Autodesk Inventor part; units mm, degrees
ref_plane "YZ Plane" through (0, 0, 0) normal (1, 0, 0) x (0, 1, 0)
ref_plane "XZ Plane" through (0, 0, 0) normal (0, 1, 0) x (-1, 0, 0)
ref_plane "XY Plane" through (0, 0, 0) normal (0, 0, 1) x (1, 0, 0)
sketch "Sketch1" plane through (0, 0, 0) normal (0, 1, 0) x (-1, 0, 0)
  line L0 (-112.5, 75) -> (112.5, 75)
  line L1 (112.5, 75) -> (112.5, -75)
  line L2 (112.5, -75) -> (-112.5, -75)
  line L3 (-112.5, -75) -> (-112.5, 75)
  line L4 (-112.5, 75) -> (112.5, -75) construction
  line L5 (112.5, 75) -> (-112.5, -75) construction
  point P0 (0, 0)
  dimension "d0" = 225
  dimension "d1" = 150
extrude "Extrusion1" add sketch "Sketch1" along normal blind 10
sketch "Sketch2" plane through (112.5, 0, 75) normal (1, 0, 0) x (0, 0, -1)
  line L0 (0, 2.5) -> (150, 2.5)
  line L1 (150, 2.5) -> (150, 7.5)
  line L2 (150, 7.5) -> (0, 7.5)
  line L3 (0, 7.5) -> (0, 2.5)
  point P0 (75, 0)
  point P1 (0, 5)
  dimension "d4" = 150
  dimension "d5" = 5
extrude "Extrusion2" add sketch "Sketch2" along normal blind 10
sketch "Sketch3" plane through (-112.5, 0, 75) normal (0, 0, 1) x (1, 0, 0)
  line L0 (0, 2.5) -> (225, 2.5)
  line L1 (225, 2.5) -> (225, 7.5)
  line L2 (225, 7.5) -> (0, 7.5)
  line L3 (0, 7.5) -> (0, 2.5)
  point P0 (112.5, 0)
  dimension "d8" = 225
  dimension "d9" = 5
extrude "Extrusion3" add sketch "Sketch3" along normal blind 10
sketch "Sketch4" plane through (-112.5, 7.5, 75) normal (0, 1, 0) x (1, 0, 0)
  line L0 (0, -10) -> (225, -10)
  line L1 (225, -10) -> (215, -10)
  line L2 (215, -10) -> (215, 0)
  line L3 (215, 0) -> (225, 0)
  line L4 (225, 0) -> (225, -10)
  line L5 (235, 150) -> (235, 0)
  line L6 (235, 0) -> (225, 0)
  line L7 (225, 0) -> (225, 10)
  line L8 (225, 10) -> (235, 10)
  line L9 (235, 10) -> (235, 0)
  point P0 (112.5, 75)
  dimension "d12" = 10
  dimension "d13" = 10
  dimension "d14" = 10
  dimension "d15" = 10
extrude "Extrusion4" cut sketch "Sketch4" against normal blind 10
properties part number "TSU_Baseplate_Male_Cut"
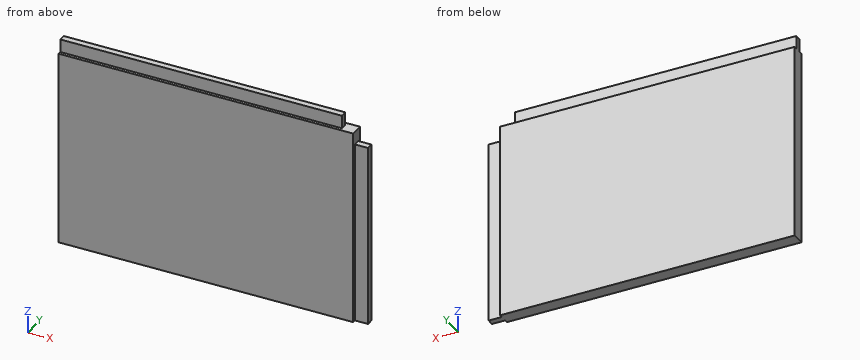
Model file for the job. Use its own axes, mm. Coordinates: 2 decimals unless noted, no trailing zeros. Loops run counter-clockwise (first coordinate to the right, second up) from the corner with the lowest first, then second, coordinate; pieces in that order, holes last. Notation, with made-up numbers: (44, 13.5) -> (57, 13.5) arc R18 ccw to (57, 17.5) -> close; hole circle Ø5 at (55.25, -24). An arc over 180 degrees is marked (long way). Use one line per item in the form item = value. Start each with the question number.
(1) Flat gauge pins, fed straight in: pin 1 (5 mm diameter, centred on x = 19.5, z = 81, fed in from -Y); pin 2 (5 mm diameter, centred on x = 118.5, z = 10, fed in from +Y); pin 3 (5.5 mm diameter, centred on x = 118.5, y = 4, fed in from +Z). Where does each tip first touch, or does it go through?
(2) Probe probe 1 along Z at (x, y) = (-2, 2); probe 2 along X at (y, z) = (4.5, 66); probe 3 along Y at (x, z) = (-65.5, 76.5). List the from-to ranges inside material, lowest first. Write a range as from..to.
(3) Cut at B-B on z = -12. Give the cut face in (x, y), and give its area (3 significant figures).
(4) Cut at A-A on x = -61.5. Give the cut face in (y, z), and give its area (3 significant figures).
Values:
q1.pin_1 = 2.5
q1.pin_2 = 7.5
q1.pin_3 = 65
q2.probe_1 = -75..75
q2.probe_2 = -112.5..112.5
q2.probe_3 = 2.5..7.5
q3.outline = (-112.5, 0) -> (112.5, 0) -> (112.5, 2.5) -> (122.5, 2.5) -> (122.5, 7.5) -> (112.5, 7.5) -> (112.5, 10) -> (-112.5, 10) -> close
q3.area = 2,300 mm2
q4.outline = (0, -75) -> (10, -75) -> (10, 75) -> (7.5, 75) -> (7.5, 85) -> (2.5, 85) -> (2.5, 75) -> (0, 75) -> close
q4.area = 1,550 mm2
